from build123d import *

# Parameters (mm, degrees)
F0_R     = 5.1
F1_DEPTH = 3
F3_DEPTH = 3
F5_D     = 3.2
F5_DEPTH = 10
F5_TIP   = 0.9613769904


with BuildPart() as f1:
    # F0 (on Front) → F1 (new body)
    with BuildSketch(Plane.XZ):
        Polygon((28, -8), (32.5, -8), (32.5, 16), (18, 16), (18, 19), (10, 19), (10, 16), (0, 16), (-10, 16), (-10, 19), (-18, 19), (-18, 16), (-32.5, 16), (-32.5, -8), (-28, -8), (-28, -11), (-20, -11), (-20, -8), (0, -8), (20, -8), (20, -11), (28, -11), align=None)
        Circle(F0_R, mode=Mode.SUBTRACT)
    extrude(amount=F1_DEPTH)

    # F2 (on face) → F3 (cut, through all)
    with BuildSketch(Plane(origin=(0, 0, 0), x_dir=(-1, 0, 0), z_dir=(0, 1, 0))):
        Polygon((13, -5), (13, -8), (16, -8), (16, -5), (17.5, -5), (17.5, -2.5), (16, -2.5), (16, -0.5), (13, -0.5), (13, -2.5), (11.5, -2.5), (11.5, -5), align=None)
        Polygon((-16, -8), (-13, -8), (-13, -5), (-11.5, -5), (-11.5, -2.5), (-13, -2.5), (-13, -0.5), (-16, -0.5), (-16, -2.5), (-17.5, -2.5), (-17.5, -5), (-16, -5), align=None)
        Polygon((26, 13), (26, 16), (23, 16), (23, 13), (21.5, 13), (21.5, 10.5), (23, 10.5), (23, 7.5), (26, 7.5), (26, 10.5), (27.5, 10.5), (27.5, 13), align=None)
        Polygon((-23, 16), (-26, 16), (-26, 13), (-27.5, 13), (-27.5, 10.5), (-26, 10.5), (-26, 7.5), (-23, 7.5), (-23, 10.5), (-21.5, 10.5), (-21.5, 13), (-23, 13), align=None)
    extrude(amount=-F3_DEPTH, mode=Mode.SUBTRACT)

    # F5
    with Locations(Plane.XZ.offset(3)):
        with Locations((-8, 0), (0, 8), (8, 0)):
            Hole(F5_D / 2, depth=F5_DEPTH)
            with Locations((0, 0, -(F5_DEPTH + F5_TIP / 2))):  # 118° drill point
                Cone(0, F5_D / 2, F5_TIP, mode=Mode.SUBTRACT)


solid = f1.part
Input: part model. Units: mm. Frame: model coordinates. A direction names the side the tool comes from. Coordinates: 2 decimals unless noted, no trailing zeros. Order: outer loops, then holes, each group sorted by start corner. A loop starts at its lowest first (then second) coordinate and runs counter-clockwise, first axis right, second up. Notation, with made-up numbers: M -26.5,68 L -18.5,68 A13 cw -18.5,91 Z; hole C 56.25,-35 d8. An arc over 180 degrees is marked long. Answer in a Markdown table with one row per item.
(1) Section query B-B, the plane z = 17. Output: boundary loops of the cut face in (x, y).
Numbers:
| item | result |
|---|---|
| outline | M -18,-3 L -10,-3 L -10,0 L -18,0 Z; M 10,-3 L 18,-3 L 18,0 L 10,0 Z |
(2) Section query D-D, the plane z = -7.25. Output: boundary loops of the cut face in (x, y), plus the area to 3 significant figures.
Numbers:
| item | result |
|---|---|
| outline | M -32.5,-3 L -16,-3 L -16,0 L -32.5,0 Z; M -13,-3 L 13,-3 L 13,0 L -13,0 Z; M 16,-3 L 32.5,-3 L 32.5,0 L 16,0 Z |
| area | 177 mm^2 |
(3) Material intervals for line 1 (X direction, y = -2.65, z = -5.5); line 2 (X direction, y = -2.4, z = 12.25); line 3 (Z direction, x = 0, y = -1.25), sorted ascending. Write a range as [from, to].
Numbers:
| item | result |
|---|---|
| line 1 | x = [-32.5, -16], [-13, 13], [16, 32.5] |
| line 2 | x = [-32.5, -27.5], [-21.5, 21.5], [27.5, 32.5] |
| line 3 | z = [-8, -5.1], [5.1, 6.4], [9.6, 16] |
(4) Section query C-C, the plane x = 0. Output: boundary loops of the cut face in (y, z), plus the area to 3 significant figures.
Numbers:
| item | result |
|---|---|
| outline | M -3,-8 L 0,-8 L 0,-5.1 L -3,-5.1 Z; M -3,5.1 L 0,5.1 L 0,6.4 L -3,6.4 Z; M -3,9.6 L 0,9.6 L 0,16 L -3,16 Z |
| area | 31.8 mm^2 |
(5) Contact query for flat-ended pins moving along their axis: pin 1 Ø8 at (x, z) = (-11.5, -6) entering from +Y; pin 2 Ø1.5 at (x, y) = (-25, -1) entering from +Z; pin 3 Ø1 at (x, y) = (17.5, -0.5) entering from -Z. Output: stop coordinate, or through.
Numbers:
| item | result |
|---|---|
| pin 1 | stops at y = 0 |
| pin 2 | stops at z = 7.5 |
| pin 3 | stops at z = -8 |
(6) Access query for faces 5 (the flat face through (-28, -1, -9)), 6 (the flat face through (18, -1, -8)), 7 (the flat face through (-23, -1, 9)), 8 (the flat face through (22, -1, 13)), 9 (the flat face through (30, -1, -8)). Directions: +Z, -Z, +X, -X, +Y, -Y. A direction counts if a zero-diameter tool reaches every point of the face in a straight line with its end or side. Return the directions, or none.
Numbers:
| item | result |
|---|---|
| face 5 | -Z, -X, +Y, -Y |
| face 6 | -Z, +Y, -Y |
| face 7 | +Z, +Y, -Y |
| face 8 | +Y, -Y |
| face 9 | -Z, +X, +Y, -Y |
(7) Draft query along X for faces 1 (the flat face through (-18, -1, 18)), 2 (the flat face through (-10, -1, 17)), 3 (the flat face through (32.5, -1, 4)), 4 (the cylindrical face through (0.35, -1.48, 6.44)). Return one class per face: pulls with the +X half, pulls with the -X half, needs draft (parallel to the pull), parting line crosses it, or undercut.
Numbers:
| item | result |
|---|---|
| face 1 | pulls with the -X half |
| face 2 | undercut |
| face 3 | pulls with the +X half |
| face 4 | undercut |
(8) Section query A-A, the plane x = 8. Output: boundary loops of the cut face in (y, z).
Numbers:
| item | result |
|---|---|
| outline | M -3,-8 L 0,-8 L 0,-1.6 L -3,-1.6 Z; M -3,1.6 L 0,1.6 L 0,16 L -3,16 Z |
